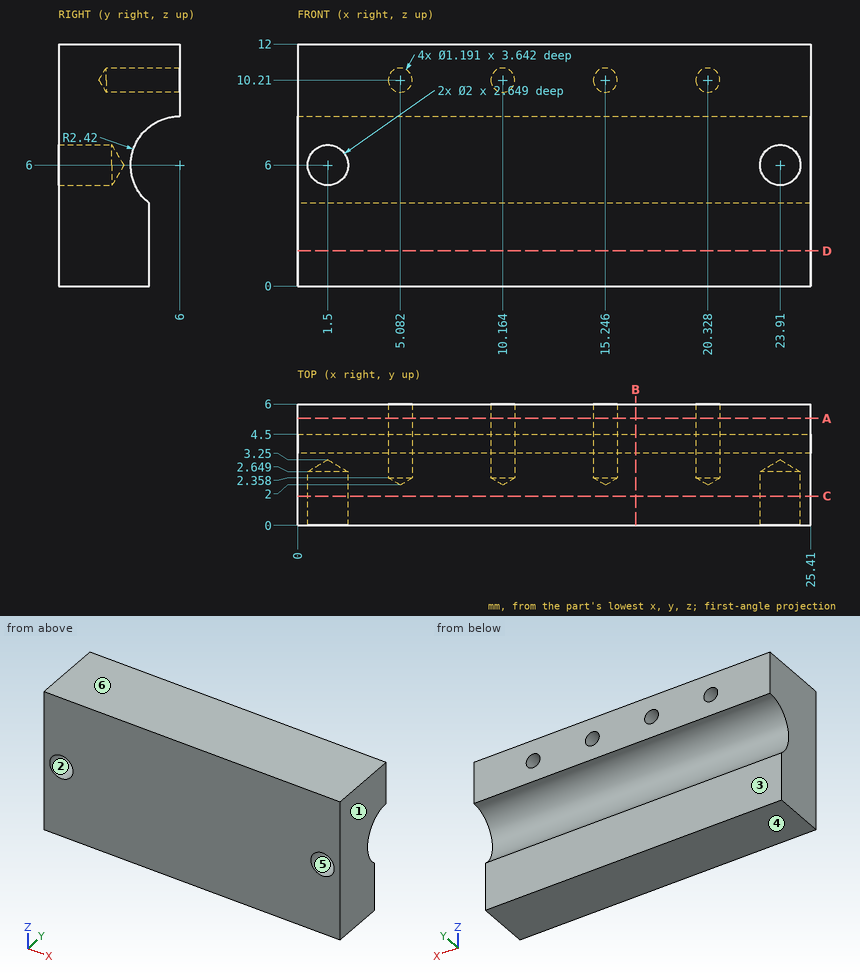
Design review of the part shown in the three views and the two pictorial views. Dimensions are in mm from the part's minimum x, y and z. A direction names the side the tool comes from. Round coordinates to 2 decimals unless told otherwise and drop trailing zeros. Loops run counter-clockwise (first coordinate to the right, second up) from the corner with the lowest first, then second, coordinate; pieces in that order, holes last. Notation, with made-up numbers: (-12.5, -4.5) - (9.5, -4.5) arc R30 ccw to (9.5, 21.5) - close; hole circle Ø4 at (12.25, 49). An arc over 180 degrees is marked (long way). Use one line per item in the form item = value.
1) We need section A-A on y = 5.3. Write out the cut boundary in (x, z).
Solutions:
outline = (0, 8.32) - (25.41, 8.32) - (25.41, 12) - (0, 12) - close; hole circle Ø1.19 at (5.08, 10.21); hole circle Ø1.19 at (10.16, 10.21); hole circle Ø1.19 at (15.25, 10.21); hole circle Ø1.19 at (20.33, 10.21)
2) We need section C-C on y = 1.45. Write out the cut boundary in (x, z), then the cut area to 3 significant figures.
Solutions:
outline = (0, 0) - (25.41, 0) - (25.41, 12) - (0, 12) - close; hole circle Ø2 at (1.5, 6); hole circle Ø2 at (23.91, 6)
area = 299 mm2
3) Tool access review of the marked faces 1, 2 and 3: name each direction out of +Z, -Z, +X, -X, +Y, -Y from which nothing blocks a thin tool from reaching the whole face with its end or side.
Solutions:
face_1 = +Z, -Z, +X, +Y, -Y
face_2 = -Y
face_3 = -Z, +X, -X, +Y
4) We need section B-B on x = 16.75. Write out the cut boundary in (y, z), then the cut area to 3 significant figures.
Solutions:
outline = (0, 0) - (4.5, 0) - (4.5, 4.1) arc R2.42 cw to (6, 8.42) - (6, 12) - (0, 12) - close
area = 57.2 mm2
5) Mouldability with a two-part tool opening along Z and no side actions: class the marked faces 4, 5 and 6 as pulls with the +Z half, pulls with the -Z half, needs draft (parallel to the pull), parting line crosses it, or undercut.
Solutions:
face_4 = pulls with the -Z half
face_5 = undercut
face_6 = pulls with the +Z half
6) Clearance check with flat-ended pins moving along their axes: P1, Ø1, axis at y = 2.5, z = 4, coming from the -X side; P2, Ø2.5, axis at x = 1.5, z = 6, coming from the +Y side; P3, Ø1.1, axis at x = 15.246, z = 10.21, coming from the +Y side; P4, Ø3.5, axis at x = 17.5, z = 1.5, coming from the +Y side. State where each tip first meets the part, or that it passes through.
Solutions:
P1 = 0
P2 = 3.93
P3 = 2.33
P4 = 4.5
7) We need section D-D on z = 1.75. Write out the cut boundary in (x, y).
Solutions:
outline = (0, 0) - (25.41, 0) - (25.41, 4.5) - (0, 4.5) - close
8) Wall thickness on probe 1 along Z at (x, y) = (1.5, 2.05); probe 2 along X at (y, z) = (3.05, 10.5) (1 decimal); probe 3 along Y at (x, z) = (2.25, 3.5): over which ranges is each line inside the solid? List them lowest first.
Solutions:
probe_1 = 0 to 5, 7 to 12
probe_2 = 0 to 4.6, 5.6 to 9.6, 10.7 to 14.7, 15.8 to 19.8, 20.8 to 25.4
probe_3 = 0 to 4.5
